Geometry: final body of the model. Coordinates: model frame, mm. A direction names the side the tool comes from. Coordinates: 2 decimals unless noted, no trailing zeros. Write each loop counter-clockwise with the first axis right and the second up, starting at its lowest first coordinate (ties: lowest second). Pieces come first, ordered by that corner, then holes. Notation, with made-up numbers: (-37.5, 36) - (-25.5, 36) arc R17 ccw to (-25.5, 55) - close; hole circle Ø1 at (27.25, 0.25). An arc over 180 degrees is marked (long way). Answer as a JSON object with one key per item and string values. Group by question number.
Item 1: Mould query, pull axis Y, two halves, no side actions, for faces 1 (the flat face through (-12.065, 4, 1)), 2 (the flat face through (-13.85, 15, 2)), 3 (the flat face through (23.85, -1, 1)), 4 (the flat face through (18, 55, 1)). Classes: pulls with the +Y half, pulls with the -Y half, needs draft (parallel to the pull), parting line crosses it, or undercut.
Item 2: Line query: line 1 along X through (y, z) = (15, 1.65); line 2 along X through (y, z) = (13.5, 1.55); line 3 along Y through (x, z) = (-10, 0.25). Output: solid intervals per line, ascending. Write a range as from..to.
Item 3: First-contact query: pin 1 Ø1.5 at (x, z) = (-11, 1.5) entering from +Y; pin 2 Ø10 at (x, y) = (-6.5, 31) entering from -Z; pin 3 Ø1.5 at (x, z) = (-12, 1.5) entering from +Y. Flat tips, straight axial feed; report the tip coordinate or a pass-through.
Item 4: Section B-B on x = 0. Return loops of the section in (y, z).
Item 5: Set-up query: faces 5 (the flat face through (0, 24.5, 1)), 6 (the flat face through (12, -17.45, 2)), 7 (the flat face through (0, -24.5, 1)). Return all of +Z, -Z, +X, -X, +Y, -Y with unobstructed straight access to the full face (end or side cutting, diameter ignored); none if empty.
Item 6: Section C-C on z = 2.25. State how many separate pieces and enclosed holes the cut face has, and give its area (3 significant figures).
Item 7: Section A-A on y = -43. Return loops of the section in (x, z).
Autodesk Inventor part; units mm, degrees
ref_plane "YZ Plane" through (0, 0, 0) normal (1, 0, 0) x (0, 1, 0)
ref_plane "XZ Plane" through (0, 0, 0) normal (0, 1, 0) x (-1, 0, 0)
ref_plane "XY Plane" through (0, 0, 0) normal (0, 0, 1) x (1, 0, 0)
sketch "草圖1" plane through (0, 0, 0) normal (0, 0, 1) x (1, 0, 0)
  line L0 (-23.85, -55) -> (23.85, 55) construction
  line L1 (23.85, -55) -> (-23.85, 55) construction
  line L2 (0, 127.5618) -> (0, -161.5218) construction
  line L3 (-23.85, 53) -> (-23.85, -53)
  line L4 (23.85, -53) -> (23.85, 53)
  line L5 (-10.5, 24.5) -> (10.5, 24.5)
  line L6 (12.5, 26.5) -> (12.5, 53)
  line L7 (-12.5, 53) -> (-12.5, 26.5)
  line L8 (-12.5, 24.5) -> (12.5, 55) construction
  line L9 (12.5, 24.5) -> (-12.5, 55) construction
  line L10 (21.85, 55) -> (14.5, 55)
  line L11 (-14.5, 55) -> (-21.85, 55)
  arc A0 (-12.5, 53) -> (-14.5, 55) centre (-14.5, 53) ccw
  arc A1 (14.5, 55) -> (12.5, 53) centre (14.5, 53) ccw
  arc A2 (-12.5, 26.5) -> (-10.5, 24.5) centre (-10.5, 26.5) ccw
  arc A3 (10.5, 24.5) -> (12.5, 26.5) centre (10.5, 26.5) ccw
  arc A4 (-21.85, 55) -> (-23.85, 53) centre (-21.85, 53) ccw
  arc A5 (23.85, 53) -> (21.85, 55) centre (21.85, 53) ccw
  line L12 (-82.8249, 0) -> (86.4934, 0) construction
  line L13 (-10.5, -24.5) -> (10.5, -24.5)
  line L14 (12.5, -26.5) -> (12.5, -53)
  line L15 (-12.5, -53) -> (-12.5, -26.5)
  line L16 (-12.5, -24.5) -> (12.5, -55) construction
  line L17 (12.5, -24.5) -> (-12.5, -55) construction
  line L18 (21.85, -55) -> (14.5, -55)
  line L19 (-14.5, -55) -> (-21.85, -55)
  arc A6 (-14.5, -55) -> (-12.5, -53) centre (-14.5, -53) ccw
  arc A7 (12.5, -53) -> (14.5, -55) centre (14.5, -53) ccw
  arc A8 (-10.5, -24.5) -> (-12.5, -26.5) centre (-10.5, -26.5) ccw
  arc A9 (12.5, -26.5) -> (10.5, -24.5) centre (10.5, -26.5) ccw
  arc A10 (-23.85, -53) -> (-21.85, -55) centre (-21.85, -53) ccw
  arc A11 (21.85, -55) -> (23.85, -53) centre (21.85, -53) ccw
  line L20 (-21.85, -55) -> (-14.5, -55)
  line L21 (14.5, -55) -> (21.85, -55)
  line L22 (-6.85, -17.45) -> (6.85, -17.45)
  line L23 (6.85, 16.75) -> (-6.85, 16.75)
  line L24 (12.065, 0.7) -> (12.065, 6.7)
  line L25 (-12.065, 6.7) -> (-12.065, 0.7)
  line L26 (-12.065, 0.7) -> (12.065, 6.7) construction
  line L27 (12.065, 0.7) -> (-12.065, 6.7) construction
  line L28 (-6.85, 16.75) -> (-6.85, 6.7)
  line L29 (6.85, 6.7) -> (6.85, 16.75)
  line L30 (12.065, 6.7) -> (6.85, 6.7)
  line L31 (7.85, 0.7) -> (12.065, 0.7)
  line L32 (-12.065, 0.7) -> (-7.85, 0.7)
  line L33 (-6.85, 6.7) -> (-12.065, 6.7)
  line L34 (-7.85, 0.7) -> (-7.85, -5.3)
  line L35 (-7.85, -5.3) -> (-6.85, -5.3)
  line L36 (-6.85, -5.3) -> (-6.85, -17.45)
  line L37 (7.85, 0.7) -> (7.85, -5.3)
  line L38 (7.85, -5.3) -> (6.85, -5.3)
  line L39 (6.85, -17.45) -> (6.85, -5.3)
  point P0 (0, 0)
  point P1 (0, 39.75)
  point P2 (0, -39.75)
  point P3 (0, 3.7)
  point P4 (12.065, 3.7)
  point P5 (-23.85, -53)
  dimension "d0" = 47.7
  dimension "d22" = 25
  dimension "d24" = 2
  dimension "d25" = 2
  dimension "d26" = 34.2
  dimension "d27" = 13.7
  dimension "d28" = 6
  dimension "d30" = 24.13
  dimension "d31" = 10.05
  dimension "d97" = 6
  dimension "d98" = 1
  dimension "d101" = 0.7
  dimension "d103" = 110
  dimension "d104" = 7.75
extrude "擠出1" add sketch "草圖1" along normal blind 3
sketch "草圖3" plane through (0, 0, 3) normal (0, 0, 1) x (1, 0, 0)
  line L0 (-88.1264, 0) -> (75.7938, 0)
  line L1 (0, 123.8394) -> (0, -129.4918)
  point P0 (0, 0)
sketch "草圖5" plane through (0, 0, 3) normal (0, 0, 1) x (1, 0, 0)
  line L0 (-9.85, -17.45) -> (-13.85, -17.45)
  line L1 (-13.85, -17.45) -> (-13.85, -14.45)
  line L2 (-13.85, -14.45) -> (-9.85, -14.45)
  line L3 (-9.85, -14.45) -> (-9.85, -17.45)
  line L4 (6.85, -17.45) -> (-6.85, -17.45)
  line L5 (-9.85, 13.75) -> (-13.85, 13.75)
  line L6 (-13.85, 13.75) -> (-13.85, 16.75)
  line L7 (-13.85, 16.75) -> (-9.85, 16.75)
  line L8 (-9.85, 16.75) -> (-9.85, 13.75)
  line L9 (-6.85, 16.75) -> (6.85, 16.75)
  line L10 (0, 31.1544) -> (0, -25.4134)
  line L11 (9.85, -17.45) -> (13.85, -17.45)
  line L12 (13.85, -17.45) -> (13.85, -14.45)
  line L13 (13.85, -14.45) -> (9.85, -14.45)
  line L14 (9.85, -14.45) -> (9.85, -17.45)
  line L15 (13.85, 16.75) -> (9.85, 16.75)
  line L16 (13.85, 13.75) -> (13.85, 16.75)
  line L17 (9.85, 13.75) -> (13.85, 13.75)
  line L18 (9.85, 16.75) -> (9.85, 13.75)
  line L19 (-17.85, 1.825) -> (-20.85, 1.825)
  line L20 (-20.85, 1.825) -> (-20.85, 13.825)
  line L21 (-20.85, 13.825) -> (-17.85, 13.825)
  line L22 (-17.85, 13.825) -> (-17.85, 1.825)
  line L23 (17.85, 1.825) -> (20.85, 1.825)
  line L24 (20.85, 1.825) -> (20.85, 13.825)
  line L25 (20.85, 13.825) -> (17.85, 13.825)
  line L26 (17.85, 13.825) -> (17.85, 1.825)
  line L27 (-6.85, -17.45) -> (-6.85, 16.75) construction
  point P0 (0, 0)
  dimension "d60" = 4
  dimension "d62" = 3
  dimension "d64" = 3
  dimension "d66" = 3
  dimension "d67" = 12
  dimension "d96" = 3
  dimension "d100" = 11
  dimension "d102" = 0.075
extrude "擠出4" cut sketch "草圖5" against normal up to next
properties part number "main_frame" material "木材 (楓木)"
Checks:
{
 "1": {"face 1": "undercut", "face 2": "undercut", "face 3": "needs draft", "face 4": "pulls with the +Y half"},
 "2": {"line 1": "-23.85..-13.85, -9.85..-6.85, 6.85..9.85, 13.85..23.85", "line 2": "-23.85..-20.85, -17.85..-6.85, 6.85..17.85, 20.85..23.85", "line 3": "-24.5..-17.45, -14.45..0.7, 6.7..13.75, 16.75..24.5"},
 "3": {"pin 1": "y = 24.94", "pin 2": "through", "pin 3": "y = 53.97"},
 "4": {"outline": "(-24.5, 0) - (-17.45, 0) - (-17.45, 3) - (-24.5, 3) - close; (16.75, 0) - (24.5, 0) - (24.5, 3) - (16.75, 3) - close"},
 "5": {"face 5": "+Z, -Z, +Y", "face 6": "+Z, -Z", "face 7": "+Z, -Z, -Y"},
 "6": {"separate pieces": "1", "enclosed holes": "7", "area": "3,060 mm^2"},
 "7": {"outline": "(-23.85, 0) - (-12.5, 0) - (-12.5, 3) - (-23.85, 3) - close; (12.5, 0) - (23.85, 0) - (23.85, 3) - (12.5, 3) - close"}
}
